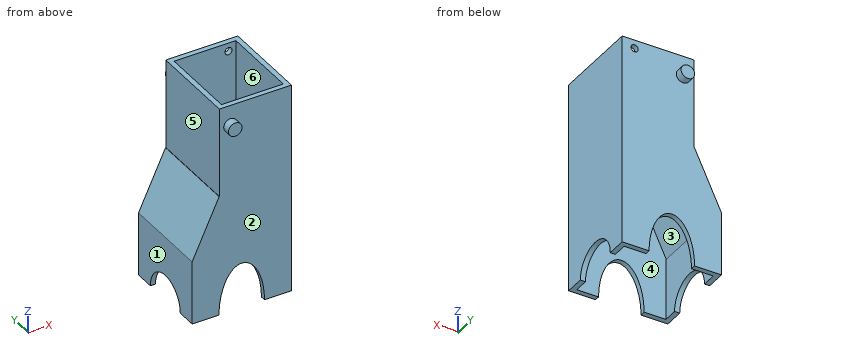
```python
from build123d import *

# Parameters (mm, degrees)
ESQUISSE1_W                 = 43.9
ESQUISSE1_H                 = 39.2
BOSS_EXTRU_1_DEPTH          = 93.38
ESQUISSE2_W                 = 12.06
ESQUISSE2_H                 = 39.7
ENL_V_MAT_EXTRU_1_DEPTH     = 93.38
ENL_V_START                 = -68.408340654
ENL_V_MAT_EXTRU_2_OUTLINE_W = 39.2
ENL_V_MAT_EXTRU_2_OUTLINE_H = 28.154614495
ENL_V_MAT_EXTRU_2_DEPTH     = 16.704392322
ESQUISSE4_W                 = 39.36
ESQUISSE4_H                 = 34.66
ENL_V_MAT_EXTRU_3_DEPTH     = 27.4
ESQUISSE5_W                 = 27.3
ESQUISSE5_H                 = 34.66
ENL_V_MAT_EXTRU_4_DEPTH     = 100
ENL_V_START_2               = -2.27
ESQUISSE6_W                 = 28.461412474
ESQUISSE6_H                 = 34.66
ENL_V_MAT_EXTRU_7_DEPTH     = 20
CONG_2_R                    = 10
ESQUISSE7_R                 = 3
BOSS_EXTRU_2_DEPTH          = 3.5
BOSS_EXTRU_3_START          = 3.5
ESQUISSE8_R                 = 3
BOSS_EXTRU_3_DEPTH          = 3.5
ESQUISSE9_R                 = 1.6
ENL_V_MAT_EXTRU_8_DEPTH     = 3.5
ESQUISSE10_RX               = 20.100105099
ESQUISSE10_RY               = 10.05
ENL_V_MAT_EXTRU_9_DEPTH     = 100
ESQUISSE12_R                = 10.95
ENL_V_MAT_EXTRU_10_DEPTH    = 100


with BuildPart() as part:
    # Esquisse1 → Boss.-Extru.1 (new body)
    with BuildSketch(Plane.XY):
        with Locations((-21.95, -19.6)):
            Rectangle(ESQUISSE1_W, ESQUISSE1_H)
    extrude(amount=BOSS_EXTRU_1_DEPTH)

    # Esquisse2 → Enlèv. mat.-Extru.1 (cut)
    with BuildSketch(Plane(origin=(0, 0, 0), x_dir=(1, 0, 0), z_dir=(0, 1, 0))):
        with Locations((-37.87, -73.53)):
            Rectangle(ESQUISSE2_W, ESQUISSE2_H)
    extrude(amount=-ENL_V_MAT_EXTRU_1_DEPTH, mode=Mode.SUBTRACT)

    # Enlèv. mat.-Extru.2: read off the stored shape, not the designer's step
    # Enlèv. mat.-Extru.2 outline → Enlèv. mat.-Extru.2 (cut)
    with BuildSketch(Plane(origin=(0, 0, 0), x_dir=(0, 1, 0), z_dir=(0.905787793342715, 0, -0.423731605419439)).offset(ENL_V_START)):
        with Locations((-19.6, 20.998682073)):
            Rectangle(ENL_V_MAT_EXTRU_2_OUTLINE_W, ENL_V_MAT_EXTRU_2_OUTLINE_H)
    extrude(amount=ENL_V_MAT_EXTRU_2_DEPTH, mode=Mode.SUBTRACT)

    # Esquisse4 → Enlèv. mat.-Extru.3 (cut)
    with BuildSketch(Plane(origin=(0, 0, 0), x_dir=(-1, 0, 0), z_dir=(0, 0, -1))):
        with Locations((21.95, -19.6)):
            Rectangle(ESQUISSE4_W, ESQUISSE4_H)
    extrude(amount=-ENL_V_MAT_EXTRU_3_DEPTH, mode=Mode.SUBTRACT)

    # Esquisse5 → Enlèv. mat.-Extru.4 (cut)
    with BuildSketch(Plane.XY.offset(93.38)):
        with Locations((-15.92, -19.6)):
            Rectangle(ESQUISSE5_W, ESQUISSE5_H)
    extrude(amount=-ENL_V_MAT_EXTRU_4_DEPTH, mode=Mode.SUBTRACT)

    # Esquisse6 → Enlèv. mat.-Extru.7 (cut)
    with BuildSketch(Plane(origin=(-46.832805267, 0, 21.908597033), x_dir=(0.42373160541943916, 0, 0.9057877933427149), z_dir=(-0.9057877933427149, 0, 0.42373160541943916)).offset(ENL_V_START_2)):
        with Locations((21.152081063, -19.6)):
            Rectangle(ESQUISSE6_W, ESQUISSE6_H)
    extrude(amount=-ENL_V_MAT_EXTRU_7_DEPTH, mode=Mode.SUBTRACT)

    # Congé2
    # the kernel refuses this fillet: 10 mm, written as the material it takes off along each edge
    with BuildSketch(Plane(origin=(-29.57, -36.93, 52.89597765), x_dir=(0, 0, 1), z_dir=(0, 1, 0))) as cong_2_piece_1:
        with BuildLine():
            CenterArc((2.157105836, -10), CONG_2_R, 90, 11.870832878)
            Line((0.10004547, -0.213861709), (0, 0))
            Line((0, 0), (2.157105836, 0))
        make_face()
    extrude(amount=34.66, mode=Mode.SUBTRACT)

    # Esquisse7 → Boss.-Extru.2 (add)
    with BuildSketch(Plane(origin=(0, -39.2, 0), x_dir=(-1, 0, 0), z_dir=(0, -1, 0))):
        with Locations((26.94, -84.38)):
            Circle(ESQUISSE7_R)
    extrude(amount=BOSS_EXTRU_2_DEPTH)

    # Esquisse8 → Boss.-Extru.3 (add)
    with BuildSketch(Plane(origin=(0, 0, 0), x_dir=(1, 0, 0), z_dir=(0, 1, 0)).offset(BOSS_EXTRU_3_START)):
        with Locations(Location((-26.94, -84.38, 0), (0, 0, 180))):
            Circle(ESQUISSE8_R)
    extrude(amount=-BOSS_EXTRU_3_DEPTH)

    # Esquisse9 → Enlèv. mat.-Extru.8 (cut)
    with BuildSketch(Plane(origin=(0, 0, 0), x_dir=(1, 0, 0), z_dir=(0, 1, 0))):
        with Locations(Location((-5.5, -89.68, 0), (0, 0, 180))):
            Circle(ESQUISSE9_R)
    extrude(amount=-ENL_V_MAT_EXTRU_8_DEPTH, mode=Mode.SUBTRACT)

    # Esquisse10 → Enlèv. mat.-Extru.9 (cut)
    with BuildSketch(Plane(origin=(0, 0, 0), x_dir=(1, 0, 0), z_dir=(0, 1, 0))):
        with Locations(Location((-21.95, 0), (0, 0, 89.814715787))):
            Ellipse(ESQUISSE10_RX, ESQUISSE10_RY)
    extrude(amount=-ENL_V_MAT_EXTRU_9_DEPTH, mode=Mode.SUBTRACT)

    # Esquisse12 → Enlèv. mat.-Extru.10 (cut)
    with BuildSketch(Plane(origin=(0, 0, 0), x_dir=(0, 0, -1), z_dir=(1, 0, 0))):
        with Locations((0, -19.6)):
            Circle(ESQUISSE12_R)
    extrude(amount=-ENL_V_MAT_EXTRU_10_DEPTH, mode=Mode.SUBTRACT)


solid = part.part
```
Geometry: final body of the model. Coordinates: model frame, mm. Face numbers are marked on the shaded views. A direction names the side the tool comes from. Coordinates: 2 decimals unless noted, no trailing zeros. Order: outer loops, then holes, each group sorted by start corner. A loop starts at its lowest first (then second) coordinate and runs counter-clockwise, first axis right, second up. Notation, with made-up numbers: (15.25, -7) -> (47.25, -7) arc R25 ccw to (47.25, 8) -> close; hole circle Ø7 at (-9.5, 65.25). An arc over 180 degrees is marked (long way). Write item = value, one per line.
(1) Cut plane D-D on z = 89.68. Return loops of the section in (x, y).
Solved:
outline = (-31.84, -39.2) -> (0, -39.2) -> (0, 0) -> (-3.9, 0) -> (-3.9, -2.27) -> (-2.27, -2.27) -> (-2.27, -36.93) -> (-29.57, -36.93) -> (-29.57, -2.27) -> (-7.1, -2.27) -> (-7.1, 0) -> (-31.84, 0) -> close
(2) Cut plane A-A on x = -10. Return loops of the section in (y, z).
Solved:
outline = (-39.2, 0) -> (-36.93, 0) -> (-36.93, 93.38) -> (-39.2, 93.38) -> close; (-2.27, 0) -> (0, 0) -> (0, 93.38) -> (-2.27, 93.38) -> close
(3) Cut plane B-B on y = -33. Return loops of the section in (x, z).
Solved:
outline = (-43.9, 0) -> (-41.63, 0) -> (-41.63, 27.12) -> (-41.84, 27.22) -> (-29.78, 53) arc R10 ccw to (-29.57, 55.05) -> (-29.57, 93.38) -> (-31.84, 93.38) -> (-31.84, 53.68) -> (-31.97, 53.68) -> (-43.9, 28.18) -> close; (-2.27, 0) -> (0, 0) -> (0, 93.38) -> (-2.27, 93.38) -> close
(4) Cut plane C-C on z = 64. Return loops of the section in (x, y), plus the area to 3 significant figures.
Solved:
outline = (-31.84, -39.2) -> (0, -39.2) -> (0, 0) -> (-31.84, 0) -> close; hole (-29.57, -36.93) -> (-2.27, -36.93) -> (-2.27, -2.27) -> (-29.57, -2.27) -> close
area = 302 mm²
(5) Pull-direction query (X, two-part tool) for the marked faces 1, 2 and 3; classes: pulls with the +X half, pulls with the -X half, needs draft (parallel to the pull), parting line crosses it, or undercut.
Solved:
face_1 = pulls with the -X half
face_2 = needs draft
face_3 = undercut
(6) Access query for the marked faces 4, 5 and 6. Directions: +Z, -Z, +X, -X, +Y, -Y. A direction counts if a zero-diameter tool reaches every point of the face in a straight line with its end or side. Return the directions, or none.
Solved:
face_4 = -Z
face_5 = +Z, -X, +Y, -Y
face_6 = +Z, -Z
(7) Pin query (flat end, axial travel): pin 1 Ø10 at (y, z) = (-5.5, 64) entering from -X; pin 2 Ø22 at (x, z) = (-19.5, 58) entering from +Y; pin 3 Ø12 at (x, z) = (-10, 10) entering from -Y; pin 4 Ø3 at (x, y) = (-25, -34.5) entering from +Z. Return the tip coordinate at first contact, or that it passes through.
Solved:
pin_1 = -31.84
pin_2 = 0
pin_3 = -39.2
pin_4 = through
(8) Line query: line 1 (X direction, y = -35, z = 72.5); line 2 (X direction, y = -8.5, z = 19.5); line 3 (Y direction, x = -9, z = 5). Output: solid intervals per line, ascending.
Solved:
line_1 = -31.84 to -29.57, -2.27 to 0
line_2 = -43.9 to -41.63, -2.27 to 0
line_3 = -39.2 to -36.93, -2.27 to 0
